Can you work these out from the drawing? Everything is in mm from the part's minimum corner. A direction names the side the tool comes from. Round coordinates to 2 decimals unless told otherwise and drop trailing zeros. Loops run counter-clockwise (first coordinate to the right, second up) from the corner with the lowest first, then second, coordinate; pieces in that order, holes last. Notation, with made-up numbers: (82, 26.5) - (123, 26.5) arc R22 ccw to (123, 44.5) - close; hole circle Ø8 at (-13, 81). An arc over 180 degrees is marked (long way). Answer as a JSON object with one key per item and string values. Group by question number.
1) If I drill on line 1 along X through (y, z) = (15, 38.5); line 2 along Y through (x, z) = (91.25, 15); line 3 along Z through (x, y) = (24, 3), over which ranges is the centre line in solid material (lowest first)? Write a range as [from, to].
2) Will these pins go through, and if not, where does the flat tip stop? P1, Ø8, axis at y = 10, z = 107, coming from the -X side; P2, Ø4, axis at x = 30.5, y = 9.5, coming from the -Z side.
3) I want a section at B-B, the plane y = 18.5. Please give me the cut outline in (x, z), then the cut area to 3 significant figures.
4) Which directions (+Z, -Z, +X, -X, +Y, -Y) give clear straight access to the entire face, cutting with the end or side of a thin tool? Please do the marked faces 1 and 2.
5) I want a section at C-C, the plane z = 15. Please give me the cut outline in (x, y).
6) I want a section at A-A, the plane z = 90.5. Please give me the cut outline in (x, y).
7) If we mould it in two halves opening along X, with no side actions, what happens to the marked faces 3, 4, 5 and 6? For each: pulls with the +X half, pulls with the -X half, needs draft (parallel to the pull), parting line crosses it, or undercut.
8) I want a section at D-D, the plane x = 31.5. Please give me the cut outline in (y, z), then the cut area to 3 significant figures.
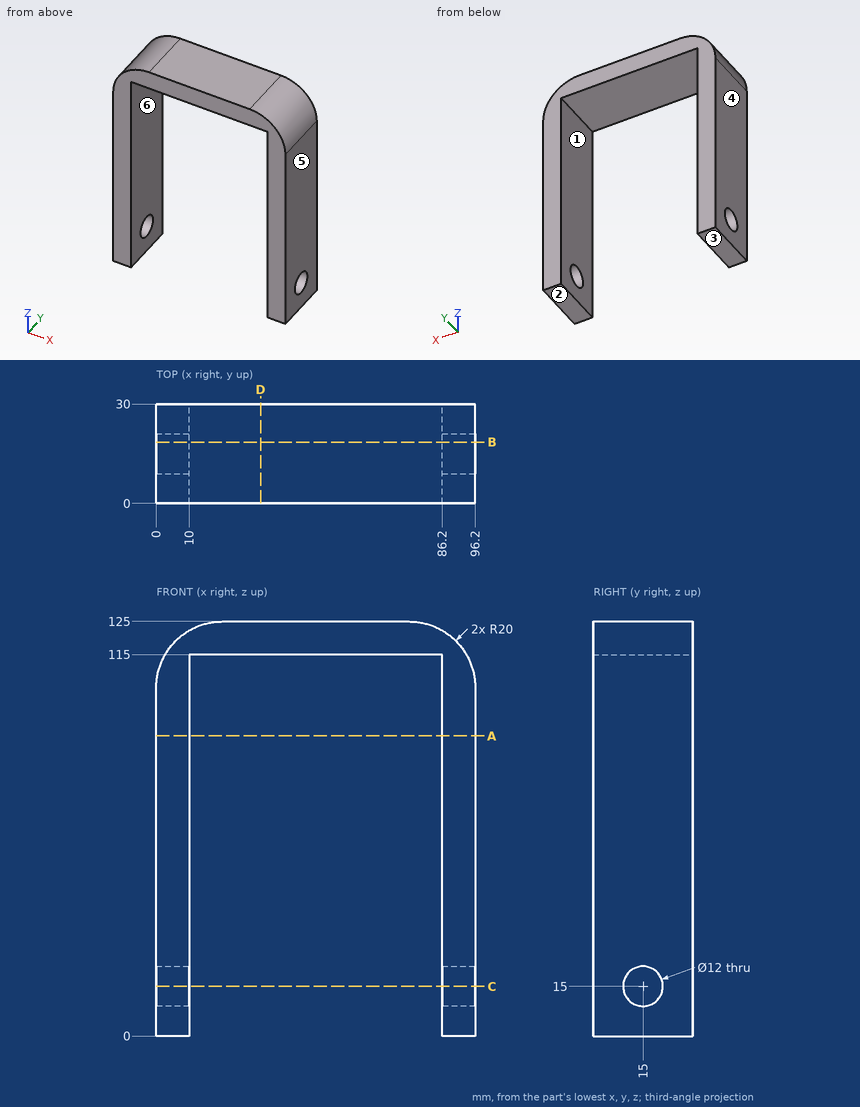
Outcome:
{
 "1": {"line 1": "[0, 10], [86.2, 96.2]", "line 2": "[0, 9], [21, 30]", "line 3": "[115, 125]"},
 "2": {"P1": "x = 0", "P2": "z = 115"},
 "3": {"outline": "(0, 0) - (10, 0) - (10, 10.13) - (0, 10.13) - close; (0, 19.87) - (10, 19.87) - (10, 115) - (86.2, 115) - (86.2, 19.87) - (96.2, 19.87) - (96.2, 105) arc R20 ccw to (76.2, 125) - (20, 125) arc R20 ccw to (0, 105) - close; (86.2, 0) - (96.2, 0) - (96.2, 10.13) - (86.2, 10.13) - close", "area": "2,900 mm^2"},
 "4": {"face 1": "-Z, +Y, -Y", "face 2": "-Z, +X, -X, +Y, -Y"},
 "5": {"outline": "(0, 0) - (10, 0) - (10, 9) - (0, 9) - close; (0, 21) - (10, 21) - (10, 30) - (0, 30) - close; (86.2, 0) - (96.2, 0) - (96.2, 9) - (86.2, 9) - close; (86.2, 21) - (96.2, 21) - (96.2, 30) - (86.2, 30) - close"},
 "6": {"outline": "(0, 0) - (10, 0) - (10, 30) - (0, 30) - close; (86.2, 0) - (96.2, 0) - (96.2, 30) - (86.2, 30) - close"},
 "7": {"face 3": "needs draft", "face 4": "pulls with the -X half", "face 5": "pulls with the +X half", "face 6": "undercut"},
 "8": {"outline": "(0, 115) - (30, 115) - (30, 125) - (0, 125) - close", "area": "300 mm^2"}
}
